Autodesk Inventor part; units mm, degrees
ref_plane "YZ Plane" through (0, 0, 0) normal (1, 0, 0) x (0, 1, 0)
ref_plane "XZ Plane" through (0, 0, 0) normal (0, 1, 0) x (-1, 0, 0)
ref_plane "XY Plane" through (0, 0, 0) normal (0, 0, 1) x (1, 0, 0)
sketch "Sketch1" plane through (0, 0, 0) normal (0, 0, 1) x (1, 0, 0)
  line L0 (-84, -25.5) -> (84, -25.5)
  line L1 (84, -25.5) -> (84, 25.5)
  line L2 (84, 25.5) -> (-84, 25.5)
  line L3 (-84, 25.5) -> (-84, -25.5)
  line L4 (-84, -25.5) -> (84, 25.5) construction
  line L5 (84, -25.5) -> (-84, 25.5) construction
  line L6 (-84, 17.5) -> (-74, 17.5)
  line L7 (-74, 17.5) -> (-74, 25.5)
  point P0 (0, 0)
  dimension "d0" = 168
  dimension "d1" = 51
  dimension "d2" = 10
  dimension "d3" = 8
extrude "Extrusion1" add sketch "Sketch1" along normal blind 9 contours L3 L6 L7 L2 L1 L0
chamfer "Chamfer1" distance 10 distance2 5 1 edges at (-84, 17.5, 4.5) measured on face at (-77.3333, 17.5, 3)
sketch "Sketch2" plane through (-84, -25.5, 0) normal (0, -1, 0) x (1, 0, 0)
  line L0 (0, 0) -> (0, 9)
  line L1 (0, 0) -> (168, 0)
  point P0 (84, 0)
  point P1 (22, 4.5)
  point P2 (42, 4.5)
  point P3 (62, 4.5)
  point P4 (82, 4.5)
  point P5 (102, 4.5)
  point P6 (122, 4.5)
  point P7 (142, 4.5)
  point P8 (162, 4.5)
  dimension "d9" = 22
  dimension "d10" = 4.5
  dimension "d13" = 20
hole "Hole1" at (-62, -25.5, 4.5) at (-42, -25.5, 4.5) at (-22, -25.5, 4.5) at (-2, -25.5, 4.5) at (18, -25.5, 4.5) at (38, -25.5, 4.5) at (58, -25.5, 4.5) direction (0, 1, 0) diameter 3 depth 10
sketch "Sketch3" plane through (0, 0, 9) normal (0, 0, 1) x (1, 0, 0)
  line L0 (-63.5, -15.5) -> (-60.5, -15.5)
  line L1 (-84, 12.5) -> (-84, -25.5)
  line L2 (-84, -15.5) -> (84, -15.5)
  line L3 (84, -25.5) -> (84, 25.5)
  line L4 (-84, 12.5) -> (-74, 17.5)
  line L5 (-84, 12.5) -> (-84, -25.5)
  line L6 (-84, -25.5) -> (84, -25.5)
  line L7 (84, -25.5) -> (84, 25.5)
  line L8 (84, 25.5) -> (-74, 25.5)
  line L9 (-74, 25.5) -> (-74, 17.5)
  line L10 (-67, 18.5) -> (77, 18.5)
  line L11 (77, 18.5) -> (77, -18.5)
  line L12 (77, -18.5) -> (-77, -18.5)
  line L13 (-77, -18.5) -> (-77, 8.1738)
  line L14 (-77, 8.1738) -> (-67, 13.1738)
  line L15 (-67, 13.1738) -> (-67, 18.5)
  line L16 (77, 18.5) -> (56.9904, -15.5) construction
  line L17 (36.9807, 18.5) -> (56.9904, -15.5) construction
  line L18 (16.9711, -15.5) -> (36.9807, 18.5) construction
  line L19 (-3.0386, 18.5) -> (16.9711, -15.5) construction
  line L20 (-23.0482, -15.5) -> (-3.0386, 18.5) construction
  line L21 (-23.0482, -15.5) -> (-43.0579, 18.5) construction
  line L22 (-63.0675, -15.5) -> (-43.0579, 18.5) construction
  line L23 (-77, 8.1738) -> (-63.0675, -15.5) construction
  line L24 (-63.5, -15.5) -> (-60.5, -15.5)
  line L25 (-63.0675, -15.5) -> (-83.0772, 18.5) construction
  line L26 (-77, 1.2732) -> (-67.1287, -15.5)
  line L27 (-73.8622, 9.7427) -> (-59.0064, -15.5)
  line L28 (-47.119, 18.5) -> (-67.1287, -15.5)
  line L29 (-38.9968, 18.5) -> (-59.0064, -15.5)
  line L30 (-47.119, 18.5) -> (-27.1094, -15.5)
  line L31 (-38.9968, 18.5) -> (-18.9871, -15.5)
  line L32 (-7.0997, 18.5) -> (-27.1094, -15.5)
  line L33 (-18.9871, -15.5) -> (1.0225, 18.5)
  line L34 (-7.0997, 18.5) -> (12.9099, -15.5)
  line L35 (1.0225, 18.5) -> (21.0322, -15.5)
  line L36 (12.9099, -15.5) -> (32.9196, 18.5)
  line L37 (41.0418, 18.5) -> (61.0515, -15.5)
  line L38 (77, 11.5994) -> (61.0515, -15.5)
  line L39 (32.9196, 18.5) -> (52.9292, -15.5)
  line L40 (41.0418, 18.5) -> (21.0322, -15.5)
  line L41 (72.9389, 18.5) -> (52.9292, -15.5)
  point P0 (0, 0)
  point P1 (-73.0724, 1.5)
  point P2 (-72.0643, -7.1134)
  point P3 (26.9759, 1.5)
  point P4 (77, -15.5)
  point P5 (-3.0386, 11.5994)
  point P6 (56.9904, -8.5994)
  point P7 (36.9807, 11.5994)
  point P8 (16.9711, -8.5994)
  point P9 (-23.0482, -8.5994)
  point P10 (-43.0579, 11.5994)
  point P11 (-77, -15.5)
  point P12 (-63.0675, -8.5994)
  dimension "d25" = 7
  dimension "d30" = 3.5
  dimension "d31" = 3.5
  dimension "d32" = 3.5
  dimension "d33" = 3.5
  dimension "d34" = 3.5
  dimension "d35" = 3.5
  dimension "d36" = 3.5
  dimension "d37" = 3.5
  dimension "d38" = 3.5
  dimension "d39" = 3.5
  dimension "d40" = 3.5
  dimension "d41" = 3.5
  dimension "d42" = 3.5
  dimension "d43" = 3.5
  dimension "d44" = 3.5
  dimension "d46" = 3.5
extrude "Extrusion2" cut sketch "Sketch3" against normal through all contours L2 L13 L26 | L29 L30 L2 | L27 L14 L15 L10 L28 | L33 L34 L2 | L31 L10 L32 | L2 L38 L11 | L40 L39 L2 | L35 L10 L36 | L37 L10 L41
fillet "Fillet1" radius 3 29 edges at (-67, 18.5, 4.5) (-67, 13.1738, 4.5) (-73.8622, 9.7427, 4.5) (-77, -15.5, 4.5) (-67.1287, -15.5, 4.5) (-43.0579, 11.5994, 4.5) (-47.119, 18.5, 4.5) (-63.0675, -8.5994, 4.5) (-59.0064, -15.5, 4.5) (-27.1094, -15.5, 4.5) (-23.0482, -8.5994, 4.5) (-38.9968, 18.5, 4.5) (-7.0997, 18.5, 4.5) (-18.9871, -15.5, 4.5) (-3.0386, 11.5994, 4.5) (12.9099, -15.5, 4.5) (16.9711, -8.5994, 4.5) (1.0225, 18.5, 4.5) (61.0515, -15.5, 4.5) (77, 11.5994, 4.5) (72.9389, 18.5, 4.5) (41.0418, 18.5, 4.5) (32.9196, 18.5, 4.5) (36.9807, 11.5994, 4.5) (21.0322, -15.5, 4.5) (52.9292, -15.5, 4.5) (56.9904, -8.5994, 4.5) (-77, 1.2732, 4.5) (77, -15.5, 4.5)
sketch "Sketch4" plane through (-74, 25.5, 0) normal (0, 1, 0) x (1, 0, 0)
  point P0 (74, 0)
sketch "Sketch5" plane through (-74, 25.5, 0) normal (0, 1, 0) x (1, 0, 0)
  line L0 (158, 0) -> (158, -9)
  line L1 (0, 0) -> (0, -9)
  line L2 (158, 0) -> (0, 0)
  line L3 (-10, 0) -> (-10, -9)
  point P0 (74, 0)
  point P1 (20.2499, -4.5)
  point P2 (60.7499, -4.5)
  point P3 (101.2499, -4.5)
  point P4 (141.7499, -4.5)
  point P5 (0, -4.5)
  dimension "d50" = 158
  dimension "d52" = 40.5
  dimension "d53" = 40.5
  dimension "d54" = 40.5
  dimension "d55" = 4.5
  dimension "d79" = 20.2499
hole "Hole2" at (-13.2501, 25.5, 4.5) at (-53.7501, 25.5, 4.5) at (27.2499, 25.5, 4.5) at (67.7499, 25.5, 4.5) direction (0, -1, 0) diameter 3 depth 10
sketch "Sketch6" plane through (0, 0, 9) normal (0, 0, 1) x (1, 0, 0)
  point P0 (0, 0)
sketch "Sketch8" plane through (-74, 25.5, 0) normal (0, 1, 0) x (1, 0, 0)
  circle A0 centre (141.7499, -4.5) radius 1.5
  circle A1 centre (101.2499, -4.5) radius 1.5
  circle A2 centre (20.2499, -4.5) radius 1.5
  circle A3 centre (60.7499, -4.5) radius 1.5
  line L0 (158, 0) -> (0, 0)
  line L1 (0, 0) -> (0, -9)
  line L2 (158, -9) -> (0, -9)
  line L3 (158, 0) -> (158, -9)
  line L4 (154, 0) -> (154, -9)
  point P0 (74, 0)
  point P1 (158, -4.5)
  point P2 (154, -4.5)
  dimension "d67" = 4
extrude "Extrusion4" [suppressed]
sketch "Sketch9" plane through (-84, -25.5, 0) normal (0, -1, 0) x (1, 0, 0)
  circle A0 centre (142, 4.5) radius 1.5
  circle A1 centre (122, 4.5) radius 1.5
  circle A2 centre (102, 4.5) radius 1.5
  circle A3 centre (82, 4.5) radius 1.5
  circle A4 centre (62, 4.5) radius 1.5
  circle A5 centre (42, 4.5) radius 1.5
  circle A6 centre (22, 4.5) radius 1.5
  line L0 (0, 0) -> (168, 0)
  line L1 (168, 0) -> (168, 9)
  line L2 (0, 9) -> (168, 9)
  line L3 (0, 0) -> (0, 9)
  point P0 (84, 0)
  point P1 (162, 4.5)
  dimension "d70" = 20
hole "Hole3" at (78, -25.5, 4.5) direction (0, 1, 0) diameter 3 depth 10
equation "\"d32\" = 0.5 * d25"
equation "\"d33\" = 0.5 * d25"
equation "\"d34\" = 0.5 * d25"
equation "\"d35\" = 0.5 * d25"
equation "\"d36\" = 0.5 * d25"
equation "\"d37\" = 0.5 * d25"
equation "\"d38\" = 0.5 * d25"
equation "\"d39\" = 0.5 * d25"
equation "\"d41\" = 0.5 * d25"
equation "\"d42\" = 0.5 * d25"
equation "\"d43\" = 0.5 * d25"
equation "\"d44\" = 0.5 * d25"
equation "\"d46\" = 0.5 * d25"
equation "\"d51\" = 0.125 * d50"
properties part number "RightTruss" material "ABS Plastic"
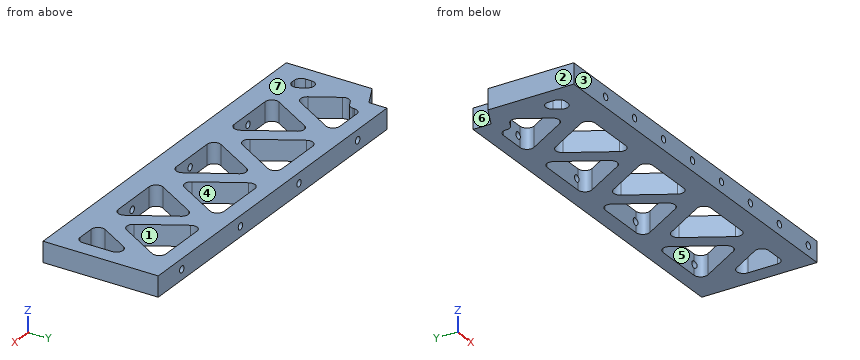
Build history of the part. All positions in model axes, mm. Face numbers are marked on the shaded views. A direction names the side the tool comes from. Round coordinates to 2 decimals unless told otherwise and drop trailing zeros. Write each loop counter-clockwise with the first axis right and the second up, starting at its lowest first coordinate (ties: lowest second). Pieces come first, ordered by that corner, then holes. Notation, with made-up numbers: M 39.5,44 L 69.5,44 A28 cw 69.5,70 Z; hole C 51,1 d2. An arc over 180 degrees is marked long. Answer in a Markdown table with one row per item.
1. Saw through at C-C (x = -62). List the corners of the cut face in (y, z).
Geometry check:
| item | result |
|---|---|
| outline | M -25.5,0 L -5.49,0 L -5.49,9 L -25.5,9 L -25.5,6 L -15.5,6 L -15.5,3 L -25.5,3 Z; M 18.5,0 L 25.5,0 L 25.5,9 L 18.5,9 Z |
2. Saw through at A-A (x = 38). List the corners of the cut face in (y, z), and give its area (3 significant figures).
Geometry check:
| item | result |
|---|---|
| outline | M -25.5,0 L -15.5,0 L -15.5,3 L -25.5,3 Z; M -25.5,6 L -15.5,6 L -15.5,9 L -25.5,9 Z; M 8.51,0 L 25.5,0 L 25.5,9 L 8.51,9 Z |
| area | 213 mm2 |
3. Flat gauge pins, fed straight in: P1, Ø1.5, axis at x = 7.5, y = 5.5, coming from the -Z side; P2, Ø0.9, axis at x = -61.5, z = 4.5, coming from the -Y side. Where does each tip first touch, or does it go through?
Geometry check:
| item | result |
|---|---|
| P1 | z = 0 |
| P2 | y = -15.5 |
4. Saw through at B-B (y = 5). State how many separate pieces and enclosed holes the cut face has, and give its area (3 significant figures).
Geometry check:
| item | result |
|---|---|
| separate pieces | 8 |
| enclosed holes | 0 |
| area | 726 mm2 |
5. Which spindle directions (+Z, -Z, +X, -X, +Y, -Y) get a long thin tool onto all of the face, cutting with end or side? Do the marked faces 5, 6 and 7. Say none if no direction does.
Geometry check:
| item | result |
|---|---|
| face 5 | +Z, -Z |
| face 6 | +Z, -Z, -X, +Y |
| face 7 | +Z, +X, -X, +Y, -Y |
6. Probe L1, parallel to Y at x = 60, z = 6.5; L2, parallel to Y at x = -32.5, z = 7; L3, parallel to Y at x = 25.5, z = 2. List the from-to ranges inside material, lowest first. Write a range as [from, to].
Geometry check:
| item | result |
|---|---|
| L1 | [-25.5, -3.49], [18.5, 25.5] |
| L2 | [-25.5, -15.5], [-6.34, 7.46], [18.5, 25.5] |
| L3 | [-25.5, -15.4], [-7.91, 5.89], [18.5, 25.5] |
7. Mould opens along Y. For the marked faces 1, 2, 3 and 4 say: +Y half, -Y half, draft (parallel to the pull), parting line (faces both ways), or undercut.
Geometry check:
| item | result |
|---|---|
| face 1 | undercut |
| face 2 | draft |
| face 3 | -Y half |
| face 4 | undercut |
